The listing builds one solid part. Answer for the finished solid, in the listing's coordinates (mm). A direction names the side the tool comes from. Give positions to 0.01 mm unless a question says otherwise; leave off trailing zeros. Write each loop counter-clockwise with the first axis right and the second up, starting at its lowest first coordinate (ties: lowest second). Pieces come first, ordered by that corner, then holes. Notation, with made-up numbers: (-18, 19) - (4, 19) arc R23 cw to (4, 31) - close; hole circle Ø8 at (13.5, 89). An arc over 180 degrees is marked (long way). Return JSON: item names as keys, results as strings.
from build123d import *

# Parameters (mm, degrees)
CROQUIS1_W              = 10
CROQUIS1_H              = 15
CROQUIS1_R              = 1.75
SALIENTE_EXTRUIR1_DEPTH = 2
CROQUIS2_W              = 10
CROQUIS2_H              = 3
SALIENTE_EXTRUIR2_DEPTH = 32
CROQUIS3_R              = 1.5
CORTAR_EXTRUIR1_DEPTH   = 36.524639337
CROQUIS4_W              = 5
CROQUIS4_H              = 10
CORTAR_EXTRUIR2_DEPTH   = 36.524639337


with BuildPart() as part:
    # Croquis1 → Saliente-Extruir1 (new body)
    with BuildSketch(Plane(origin=(0, 0, 0), x_dir=(1, 0, 0), z_dir=(0, 1, 0))):
        Rectangle(CROQUIS1_W, CROQUIS1_H)
        with Locations(Location((0, 5, 0), (0, 0, 270))):
            Circle(CROQUIS1_R, mode=Mode.SUBTRACT)
        with Locations(Location((0, -5, 0), (0, 0, 270))):
            Circle(CROQUIS1_R, mode=Mode.SUBTRACT)
    extrude(amount=SALIENTE_EXTRUIR1_DEPTH)

    # Croquis2 → Saliente-Extruir2 (add)
    with BuildSketch(Plane(origin=(0, 2, 0), x_dir=(1, 0, 0), z_dir=(0, 1, 0))):
        Rectangle(CROQUIS2_W, CROQUIS2_H)
    extrude(amount=SALIENTE_EXTRUIR2_DEPTH)

    # Croquis3 → Cortar-Extruir1 (cut, through all)
    with BuildSketch(Plane.XY.offset(1.5)):
        with Locations((0, 31)):
            Circle(CROQUIS3_R)
        with Locations((0, 12)):
            Circle(CROQUIS3_R)
    extrude(amount=-CORTAR_EXTRUIR1_DEPTH, mode=Mode.SUBTRACT)

    # Croquis4 → Cortar-Extruir2 (cut, through all)
    with BuildSketch(Plane.XY.offset(1.5)):
        with Locations((0, 21.5)):
            Rectangle(CROQUIS4_W, CROQUIS4_H)
    extrude(amount=-CORTAR_EXTRUIR2_DEPTH, mode=Mode.SUBTRACT)


solid = part.part
Item 1: The mould has two halves that part along Y. Classify faces 1 (the face through (0, 1, 7.5)), 2 (the face through (-1.11, 32.01, 0.02)), 3 (the face through (0, 2, -3)), 4 (the face through (-2.5, 21, 0)): +Y half, -Y half, draft (parallel to the pull), parting line (faces both ways), or undercut.
Answer below:
{"face 1": "draft", "face 2": "undercut", "face 3": "+Y half", "face 4": "undercut"}
Item 2: A cutting plane is placed at C-C on x = 3.75. Determine the outline of the cut face in (y, z), then the cut area to 3 significant figures.
Answer below:
{"outline": "(0, -7.5) - (2, -7.5) - (2, -1.5) - (34, -1.5) - (34, 1.5) - (2, 1.5) - (2, 7.5) - (0, 7.5) - close", "area": "126 mm²"}
Item 3: Consider L1, parallel to X at y = 21.5, z = 0; L2, parallel to X at y = 0.8, z = -5; L3, parallel to Y at x = -0.25, z = 0.5. Determine where each line is inside the solid, lowest interval first.
Answer below:
{"L1": "x = -5 to -2.5, 2.5 to 5", "L2": "x = -5 to -1.75, 1.75 to 5", "L3": "y = 0 to 10.52, 13.48 to 16.5, 26.5 to 29.52, 32.48 to 34"}
Item 4: For faces 5 (the face through (0, 26.5, 0)), 6 (the face through (0, 14, -1.5)), 7 (the face through (0, 14, 1.5)), determine the directions among +Z, -Z, +X, -X, +Y, -Y from which every point of the face is accessible in a straight line to the end or side of a thin tool.
Answer below:
{"face 5": "+Z, -Z", "face 6": "-Z, +X, -X, +Y", "face 7": "+Z, +X, -X, +Y"}
Item 5: Flat-ended cylindrical pins translate along their axes: P1, Ø3, axis at x = -1, z = -4.5, coming from the +Y side; P2, Ø2.5, axis at x = 0, y = 12, coming from the +Z side; P3, Ø4, axis at x = 2.5, z = -5, coming from the -Y side; P4, Ø6, axis at x = -3.5, y = 6.5, coming from the +Z side. Find the tip coordinate at first contact, or state that the pin passes through.
Answer below:
{"P1": "stops at y = 2", "P2": "passes through", "P3": "stops at y = 0", "P4": "stops at z = 1.5"}
Item 6: A cutting plane is placed at D-D on z = 0.5. Determine the outline of the cut face in (x, y).
Answer below:
{"outline": "(-5, 0) - (5, 0) - (5, 34) - (-5, 34) - close; hole (-2.5, 16.5) - (2.5, 16.5) - (2.5, 26.5) - (-2.5, 26.5) - close; hole circle Ø3 at (0, 12); hole circle Ø3 at (0, 31)"}
Item 7: A cutting plane is placed at B-B on y = 12. Determine the outline of the cut face in (x, z).
Answer below:
{"outline": "(-5, -1.5) - (-1.5, -1.5) - (-1.5, 1.5) - (-5, 1.5) - close; (1.5, -1.5) - (5, -1.5) - (5, 1.5) - (1.5, 1.5) - close"}
Item 8: A cutting plane is placed at A-A on z = 5. Determine the outline of the cut face in (x, y), then the cut area to 3 significant figures.
Answer below:
{"outline": "(-5, 0) - (-1.75, 0) - (-1.75, 2) - (-5, 2) - close; (1.75, 0) - (5, 0) - (5, 2) - (1.75, 2) - close", "area": "13.0 mm²"}
